from build123d import *

# Parameters (mm, degrees)
BOSS_EXTRUDE1_DEPTH = 14.1478
SKETCH2_R           = 2.9591
CUT_EXTRUDE1_DEPTH  = 14.1478


with BuildPart() as part:
    # Sketch1 → Boss-Extrude1 (new body)
    with BuildSketch(Plane.XY):
        with BuildLine():
            Line((-5.4102, 0), (-5.4102, -0.254))
            add(Edge.make_bspline(
                [(-5.4102, -0.254), (6.345e-06, -6.451600503), (5.4102, -0.254)],
                knots=[0, 0, 0, 1, 1, 1], degree=2))
            Line((5.4102, -0.254), (5.4102, 0))
            Line((5.4102, 0), (-5.4102, 0))
        make_face()
    extrude(amount=BOSS_EXTRUDE1_DEPTH)

    # Sketch2 → Cut-Extrude1 (cut)
    with BuildSketch(Plane(origin=(0, 0, 0), x_dir=(1, 0, 0), z_dir=(0, 1, 0))):
        with Locations((0, -7.0739)):
            Circle(SKETCH2_R)
    extrude(amount=-CUT_EXTRUDE1_DEPTH, mode=Mode.SUBTRACT)


solid = part.part
The model under review builds one solid part; all positions refer to its coordinate system, in mm. Give positions to 0.01 mm unless a question says otherwise; leave off trailing zeros. Answer in a Markdown table with one row per item. Add a question column.
1. To check wall thickness, follow line 1 along Z through (x, y) = (0, -2.35); line 2 along Z through (x, y) = (2, -2.5); line 3 along X through (y, z) = (-1.5, 7.5). State the ranges of each line that lie inside material, in increasing order.
2. Mouldability with a two-part tool opening along X and no side actions: class faces 1 (the cylindrical face through (-0.641, -1.28, 9.963)), 2 (the flat face through (0.1, 0, 3.8)) as released by +X, released by -X, zero draft, split by the parting line, or undercut.
3. For pin 1 Ø1 at (y, z) = (-2, 10) entering from +X; pin 2 Ø5 at (x, z) = (-1, 7) entering from +Y; pin 3 Ø1.5 at (x, z) = (-3.5, 9.5) entering from -Y, all flat-tipped, find the tip position at first contact; note any pin that passes through.
The answers:
| question | item | result |
|---|---|---|
| 1 | line 1 | 0 to 4.11, 10.03 to 14.15 |
| 1 | line 2 | 0 to 4.89, 9.25 to 14.15 |
| 1 | line 3 | -4.18 to -2.93, 2.93 to 4.18 |
| 2 | face 1 | undercut |
| 2 | face 2 | zero draft |
| 3 | pin 1 | x = 4.18 |
| 3 | pin 2 | y = 0 |
| 3 | pin 3 | y = -2.55 |
